from build123d import *

# Parameters (mm, degrees)
F2_DEPTH = 5
F3_D     = 5
F6_DEPTH = 31.3


with BuildPart() as f2:
    # F1 (on Top) → F2 (new body)
    with BuildSketch(Plane.XY):
        with BuildLine():
            ThreePointArc((-18.9928135453, 17.7327254881), (-15.4959787625, 14.226407891), (-11.9928192496, 17.726406465))
            ThreePointArc((-11.9928192496, 17.726406465), (-13.0164454835, 20.1997792575), (-15.4885752329, 21.2264038919))
            ThreePointArc((-15.4885752329, 21.2264038919), (-17.9639555673, 20.2050119801), (-18.9928135453, 17.7327254881))
        make_face()
        with BuildLine():
            ThreePointArc((-15.4885752329, 21.2264038919), (-13.0164454835, 20.1997792575), (-11.9928192496, 17.726406465))
            ThreePointArc((-11.9928192496, 17.726406465), (-15.4959787625, 14.226407891), (-18.9928135453, 17.7327254881))
            Line((-18.9928135453, 17.7327254881), (-25.4770891107, -37.888429023))
            ThreePointArc((-25.4770891107, -37.888429023), (-21.797650123, -34.7996028161), (-18.5006331801, -38.2937118411))
            ThreePointArc((-18.5006331801, -38.2937118411), (-19.4711098532, -40.7127016589), (-21.8443541735, -41.7902210821))
            Line((-21.8443541735, -41.7902210821), (21.9980642511, -41.7891520748))
            ThreePointArc((21.9980642511, -41.7891520748), (19.3836869362, -35.9620342294), (25.4744262299, -37.8837953968))
            Line((25.4744262299, -37.8837953968), (18.9895786755, 17.7319920337))
            ThreePointArc((18.9895786755, 17.7319920337), (13.0143403088, 15.2593596765), (15.4887358258, 21.2338681198))
            Line((15.4887358258, 21.2338681198), (-15.4885752329, 21.2264038919))
        make_face()
        with BuildLine():
            ThreePointArc((18.9895791784, 17.7338682214), (17.9641547244, 20.2090401077), (15.4887358258, 21.2338681198))
            ThreePointArc((15.4887358258, 21.2338681198), (13.0143403088, 15.2593596765), (18.9895786755, 17.7319920337))
            ThreePointArc((18.9895786755, 17.7319920337), (18.9895790527, 17.7329301275), (18.9895791784, 17.7338682214))
        make_face()
        with BuildLine():
            ThreePointArc((-18.5006331801, -38.2937118411), (-21.797650123, -34.7996028161), (-25.4770891107, -37.888429023))
            ThreePointArc((-25.4770891107, -37.888429023), (-24.6661333689, -40.5619950562), (-22.1567416762, -41.790228699))
            Line((-22.1567416762, -41.790228699), (-21.8443541735, -41.7902210821))
            ThreePointArc((-21.8443541735, -41.7902210821), (-19.4711098532, -40.7127016589), (-18.5006331801, -38.2937118411))
        make_face()
        with BuildLine():
            Line((-21.8443541735, -41.7902210821), (-22.1567416762, -41.790228699))
            ThreePointArc((-22.1567416762, -41.790228699), (-22.0005478398, -41.7937118401), (-21.8443541735, -41.7902210821))
        make_face()
        with BuildLine():
            ThreePointArc((25.4979789108, -38.2891520759), (25.4920857793, -38.0861319007), (25.4744262299, -37.8837953968))
            ThreePointArc((25.4744262299, -37.8837953968), (19.3836869362, -35.9620342294), (21.9980642511, -41.7891520748))
            ThreePointArc((21.9980642511, -41.7891520748), (24.4728828171, -40.7639956375), (25.4979789108, -38.2891520759))
        make_face()
    extrude(amount=F2_DEPTH)

    # F3 (through all)
    with Locations(Plane(origin=(0, 0, 0), x_dir=(1, 0, 0), z_dir=(0, 0, -1))):
        with Locations((-15.5, -17.7061764002), (15.5, -17.7061764002), (-22, 38.2938235998), (22, 38.2938235998)):
            Hole(F3_D / 2)

    # F5 (on offset) → F6 (join)
    with BuildSketch(Plane.YZ.offset(15.5)):
        Polygon((-28.8004414439, 3.5987684969), (-32.7974634149, 33.0814354707), (-37.2756377012, 40.8378608596), (-31.8004414439, 3.5987684969), align=None)
        Polygon((-37.2756377012, 40.8378608596), (-32.7974634149, 33.0814354707), (-15.7756377012, 3.5987684969), (13.7907450582, 20.6689275419), (16.9883244112, 22.5150508422), (21.4634546616, 25.0987684969), (-0.0365453384, 62.3378608596), align=None)
        Polygon((18.1931839084, 25.9461292587), (-14.7157814354, 6.9461292587), (-33.7157814354, 39.8550946025), (-0.8068160916, 58.8550946025), align=None, mode=Mode.SUBTRACT)
        Polygon((16.9883244112, 22.5150508422), (13.7907450582, 20.6689275419), (6.5782903694, 5.0800526515), (9.5782903694, 5.0800526515), align=None)
    extrude(amount=-F6_DEPTH)


solid = f2.part
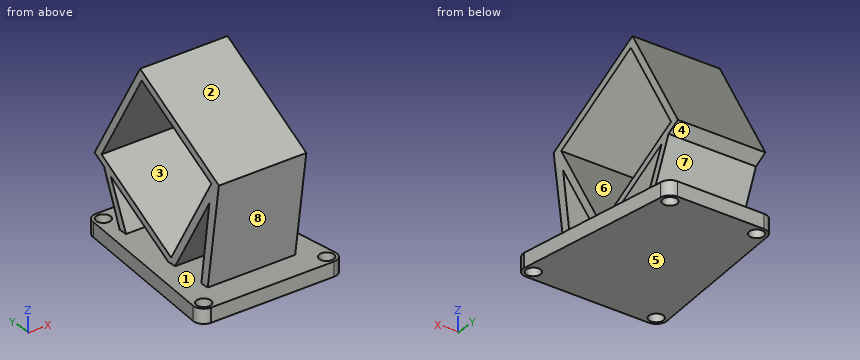
Verification items for the finished model (mm, model axes). Face numbers are marked on the shaded views. A direction names the side the tool comes from. Give positions to 0.01 mm unless a question says otherwise; leave off trailing zeros. Write each loop counter-clockwise with the first axis right and the second up, starting at its lowest first coordinate (ties: lowest second). Pieces come first, ordered by that corner, then holes. Notation, with made-up numbers: (89.25, -29) - (106.25, -29) arc R20 ccw to (106.25, 0) - close; hole circle Ø7 at (77.25, 61). An arc over 180 degrees is marked (long way). Answer as CSV lines item,"result". Start each with the question number.
1. Sectioned sample at D-D (z = 13.5). Record the boundary of the cut face in (x, y).
2. Depth check by flat-ended pin: pin 1 (8 mm diameter, centred on x = 5.5, z = 27, fed in from +Y); pin 2 (4.5 mm diameter, centred on x = -22, y = -38.29, fed in from +Z); pin 3 (2.5 mm diameter, centred on x = 0.5, z = 1.5, fed in from +Y); pin 4 (8 mm diameter, centred on x = -2, z = 50, fed in from -Y). Enter the tip coordinate at first touch or a pass-through.
3. Set-up check for the marked faces 5, 6, 7 and 8: record each of +Z, -Z, +X, -X, +Y, -Y from which the full face is reachable in a straight line by a thin tool's end or side.
4. Sectioned sample at C-C (z = 54). Record the boundary of the cut face in (x, y).
5. Sectioned sample at B-B (x = -14.5). Record the boundary of the cut face in (y, z), then the cut area to 3 significant figures.
6. Sectioned sample at A-A (y = -26). Record the boundary of the cut face in (x, z).
7. Thickness scan on line 1 (Y direction, x = -15.5, z = 3.25); line 2 (Z direction, x = 0, y = 18); line 3 (Y direction, x = 15, z = 32.5). Record the ranges inside material, lowest first.
8. Draft check along Y on the marked faces 1, 2, 3 and 4. Enter one of: pulls with the +Y half, pulls with the -Y half, needs draft (parallel to the pull), parting line crosses it, or undercut.
Derived:
1,outline,"(-15.8, -33.26) - (15.5, -33.26) - (15.5, -30.14) - (-15.8, -30.14) - close; (-15.8, -21.49) - (15.5, -21.49) - (15.5, -18.5) - (-15.8, -18.5) - close; (-15.8, -3.36) - (15.5, -3.36) - (15.5, 1.37) - (-15.8, 1.37) - close; (-15.8, 10.47) - (15.5, 10.47) - (15.5, 13.16) - (-15.8, 13.16) - close"
2,pin 1,"y = 21.46"
2,pin 2,"through"
2,pin 3,"y = 21.23"
2,pin 4,"y = -28.33"
3,face 5,"-Z, +X, -X, +Y, -Y"
3,face 6,"+X, -X"
3,face 7,"+X, -X, +Y"
3,face 8,"+X, -X, -Y"
4,outline,"(-15.8, -14.48) - (15.5, -14.48) - (15.5, -9.22) - (-15.8, -9.22) - close; (-15.8, 2) - (15.5, 2) - (15.5, 4.78) - (-15.8, 4.78) - close"
5,outline,"(-41.79, 0) - (15.41, 0) - (15.41, 5) - (-13.35, 5) - (13.79, 20.67) - (6.58, 5.08) - (9.58, 5.08) - (16.99, 22.52) - (21.46, 25.1) - (-0.04, 62.34) - (-37.28, 40.84) - (-32.01, 5) - (-41.79, 5) - close; (20, 0) - (21.23, 0) - (21.23, 5) - (20, 5) - close; hole (-33.72, 39.86) - (-14.72, 6.95) - (18.19, 25.95) - (-0.81, 58.86) - close; hole (-32.8, 33.08) - (-28.99, 5) - (-16.58, 5) - close"
5,area,"841 mm²"
6,outline,"(-24.09, 0) - (24.09, 0) - (24.09, 5) - (-24.09, 5) - close; (-15.8, 21.31) - (15.5, 21.31) - (15.5, 26.49) - (-15.8, 26.49) - close; (-15.8, 44.31) - (15.5, 44.31) - (15.5, 47.35) - (-15.8, 47.35) - close"
7,line 1,"-41.79 to 15.21, 20.21 to 21.23"
7,line 2,"0 to 5, 23.1 to 25.83, 26.28 to 31.1"
7,line 3,"-36.05 to -32.72, -32.46 to -29.47, 14.41 to 17.19"
8,face 1,"undercut"
8,face 2,"pulls with the -Y half"
8,face 3,"undercut"
8,face 4,"pulls with the +Y half"
